from build123d import *

# Parameters (mm, degrees)
F4_DEPTH = 4.5
F5_W     = 3
F5_H     = 1.5
F7_R     = 1.5
F8_DEPTH = 4.5
F9_R     = 5


with BuildPart() as f4:
    # F3 (on Top) → F4 (new body)
    with BuildSketch(Plane.XY):
        Polygon((0, -10), (0, 0), (40, 0), (40, 8), (-8, 8), (-8, -10), align=None)
    extrude(amount=F4_DEPTH)

    # F6: sweep along a path in F6_path
    with BuildLine(Plane(origin=(0, 0, 4.5), x_dir=(0, -1, 0), z_dir=(0, 0, -1))) as f6_path:
        Line((0, -40), (0, 0))
        Line((0, 0), (10, 0))
    # F5 (on face) → F6 (sweep, cut)
    with BuildSketch(Plane.YZ.offset(40)):
        with Locations((1.5, 3.75)):
            Rectangle(F5_W, F5_H)
    sweep(path=f6_path.line, transition=Transition.RIGHT, mode=Mode.SUBTRACT)

    # F7 (on face) → F8 (cut, through all)
    with BuildSketch(Plane.XY.offset(4.5)):
        with Locations((-5.5, -3.5)):
            Circle(F7_R)
        with BuildLine():
            Line((7.5, 3.9999998055), (17.5, 3.9999998055))
            ThreePointArc((17.5, 3.9999998055), (19, 5.4999998055), (17.5, 6.9999998055))
            Line((17.5, 6.9999998055), (7.5000000583, 7.0000001945))
            ThreePointArc((7.5000000583, 7.0000001945), (5.9999998055, 5.5000000292), (7.5, 3.9999998055))
        make_face()
        with Locations((22.5, 5.5)):
            Circle(F7_R)
        with BuildLine():
            Line((27.5, 4), (37.5, 4))
            ThreePointArc((37.5, 4), (39, 5.5), (37.5, 7))
            Line((37.5, 7), (27.5, 7))
            ThreePointArc((27.5, 7), (26, 5.5), (27.5, 4))
        make_face()
    extrude(amount=-F8_DEPTH, mode=Mode.SUBTRACT)

    # F9
    f9_edges = [f4.edges().sort_by_distance(p)[0] for p in [
        (-8, 8, 2.25),
    ]]
    fillet(f9_edges, radius=F9_R)


solid = f4.part
CAD build for the part. Positions are in the model's coordinates, mm. A direction names the side the tool comes from. Give positions to 0.01 mm unless a question says otherwise; leave off trailing zeros. Order: outer loops, then holes, each group sorted by start corner. A loop starts at its lowest first (then second) coordinate and runs counter-clockwise, first axis right, second up. Notation, with made-up numbers: (49.5, -15.75) -> (54.5, -15.75) arc R25 cw to (54.5, 2.25) -> close; hole circle Ø2 at (28.5, -38). An arc over 180 degrees is marked (long way). Return JSON: item names as keys, results as strings.
Q1. Drill centre lines: line 1 (Y direction, x = 15.5, z = 2.2); line 2 (X direction, y = -8, z = 4.15); line 3 (Z direction, x = 14.5, y = 1.75). Where is each one in solid material? Low to high.
Working result:
{"line 1": "0 to 4, 7 to 8", "line 2": "-8 to -3", "line 3": "0 to 3"}
Q2. Saw through at C-C (z = 1.85). Write the cut outline in (x, y), then the cut area to 3 significant figures.
Working result:
{"outline": "(-8, -10) -> (0, -10) -> (0, 0) -> (40, 0) -> (40, 8) -> (-3, 8) arc R5 ccw to (-8, 3) -> close; hole circle Ø3 at (-5.5, -3.5); hole (7.5, 4) -> (17.5, 4) arc R1.5 ccw to (17.5, 7) -> (7.5, 7) arc R1.5 ccw to start; hole circle Ø3 at (22.5, 5.5); hole (27.5, 4) -> (37.5, 4) arc R1.5 ccw to (37.5, 7) -> (27.5, 7) arc R1.5 ccw to start", "area": "370 mm²"}
Q3. Flat gauge pins, fed straight in: pin 1 (2.5 mm diameter, centred on x = -5.5, y = -3.5, fed in from +Z); pin 2 (1.6 mm diameter, centred on x = 8, z = 3.5, fed in from -Y); pin 3 (1.5 mm diameter, centred on y = -7, z = 2, fed in from +X). Where does each tip first touch, or does it go through?
Working result:
{"pin 1": "through", "pin 2": "y = 0", "pin 3": "x = 0"}
Q4. Mould opens along X. For faces 1 (the face through (-7, 6, 2)), 2 (the face through (6, 5.5, 2.3)), 3 (the face through (10, 1, 0)) say: pulls with the +X half, pulls with the -X half, needs draft (parallel to the pull), parting line crosses it, or undercut.
Working result:
{"face 1": "pulls with the -X half", "face 2": "undercut", "face 3": "needs draft"}
Q5. Saw through at A-A (y = -3.5). Write the cut outline in (x, z), then the cut area to 3 significant figures.
Working result:
{"outline": "(-8, 0) -> (-7, 0) -> (-7, 4.5) -> (-8, 4.5) -> close; (-4, 0) -> (0, 0) -> (0, 3) -> (-3, 3) -> (-3, 4.5) -> (-4, 4.5) -> close", "area": "18.0 mm²"}
Q6. Saw through at D-D (y = 6.5). Write the cut outline in (x, z).
Working result:
{"outline": "(-6.57, 0) -> (6.38, 0) -> (6.38, 4.5) -> (-6.57, 4.5) -> close; (18.62, 0) -> (21.38, 0) -> (21.38, 4.5) -> (18.62, 4.5) -> close; (23.62, 0) -> (26.38, 0) -> (26.38, 4.5) -> (23.62, 4.5) -> close; (38.62, 0) -> (40, 0) -> (40, 4.5) -> (38.62, 4.5) -> close"}
Q7. Which spindle directions (+Z, -Z, +X, -X, +Y, -Y) get a long thin tool onto all of the face, cutting with end or side? Do faces 4 (the face through (20, 0, 1)), 5 (the face through (15.4, 0.3, 3)), 6 (the face through (8.8, 3.7, 4.5)), 7 (the face through (12, 4, 2)), 8 (the face through (19, 8, 2)). Say none if no direction does.
Working result:
{"face 4": "+Z, -Z, +X, -Y", "face 5": "+Z, +X, -Y", "face 6": "+Z, +X, -X, +Y, -Y", "face 7": "+Z, -Z", "face 8": "+Z, -Z, +X, -X, +Y"}
Q8. Saw through at B-B (x = 29). Write the cut outline in (y, z), then the cut area to 3 significant figures.
Working result:
{"outline": "(0, 0) -> (4, 0) -> (4, 4.5) -> (3, 4.5) -> (3, 3) -> (0, 3) -> close; (7, 0) -> (8, 0) -> (8, 4.5) -> (7, 4.5) -> close", "area": "18.0 mm²"}
